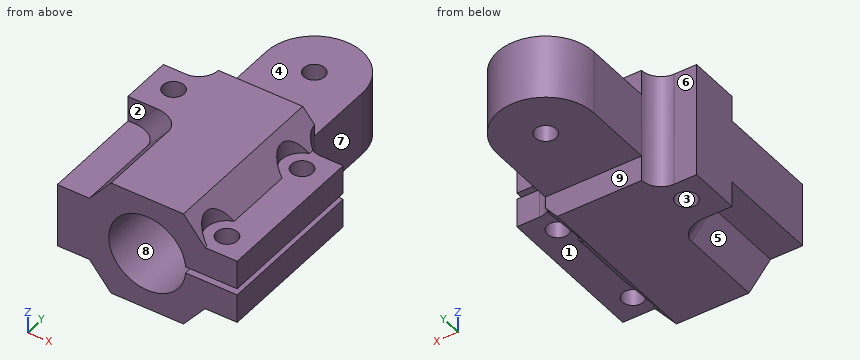
from build123d import *

# Parameters (mm, degrees)
F2_DEPTH        = 9
F3_R            = 6
F4_DEPTH        = 24
F6_DEPTH        = 45.3215080757
F7_DEPTH        = 16
F8_R            = 3
F10_DEPTH       = 21.501
F12_D           = 3.3
F12_START       = 4
F12_CBORE_D     = 6.5
F12_CBORE_DEPTH = 0
F14_D           = 3.3
F14_START       = 4
F14_CBORE_D     = 6.5
F14_CBORE_DEPTH = 0
F15_W           = 27
F15_H           = 1
F16_DEPTH       = 30


with BuildPart() as f2:
    # F1 (on Top) → F2 (new body, symmetric)
    with BuildSketch(Plane.XY):
        with BuildLine():
            ThreePointArc((-7.5, 0), (0, -7.5), (7.5, 0))
            ThreePointArc((7.5, 0), (0, 7.5), (-7.5, 0))
        make_face()
        with BuildLine():
            Line((7.5, -13.8205080757), (7.5, 0))
            ThreePointArc((7.5, 0), (0, -7.5), (-7.5, 0))
            Line((-7.5, 0), (-7.5, -13.8205080757))
            Line((-7.5, -13.8205080757), (-14, -13.8205080757))
            Line((-14, -13.8205080757), (-14, -37.8205080757))
            Line((-14, -37.8205080757), (14, -37.8205080757))
            Line((14, -37.8205080757), (14, -13.8205080757))
            Line((14, -13.8205080757), (7.5, -13.8205080757))
        make_face()
    extrude(amount=F2_DEPTH, both=True)

    # F3 (on face) → F4 (cut)
    with BuildSketch(Plane.XZ.offset(37.8205080757)):
        Circle(F3_R)
    extrude(amount=-F4_DEPTH, mode=Mode.SUBTRACT)

    # F5 (on face) → F6 (cut, through all)
    with BuildSketch(Plane.XZ.offset(37.8205080757)):
        Polygon((14, 9), (5.6436014753, 9), (9, 5), (14, 5), align=None)
        Polygon((14, -9), (14, -5), (9, -5), (5.6436014753, -9), align=None)
    extrude(amount=-F6_DEPTH, mode=Mode.SUBTRACT)

    # F5 (on face) → F7 (cut)
    with BuildSketch(Plane.XZ.offset(37.8205080757)):
        Polygon((-9, 5), (-5.6436014753, 9), (-14, 9), (-14, 5), align=None)
        Polygon((-9, -5), (-14, -5), (-14, -9), (-5.6436014753, -9), align=None)
    extrude(amount=-F7_DEPTH, mode=Mode.SUBTRACT)

    # F8
    f8_edges = [f2.edges().sort_by_distance(p)[0] for p in [
        (7.5, -13.820508, 0),
        (-7.5, -13.820508, 0),
        (-7.321801, -21.820508, 7),
        (-7.321801, -21.820508, -7),
    ]]
    fillet(f8_edges, radius=F8_R)

    # F9 (on face) → F10 (cut, through all)
    with BuildSketch(Plane.YZ.offset(7.5)):
        Polygon((9.9274870008, 9), (4.9396115625, 9), (-10.8205080757, 9), (-10.8205080757, 6.7876303889), (-10.8205080757, 5), (9.9274870008, 5), align=None)
        Polygon((9.9274870008, -5), (-10.8205080757, -5), (-10.8205080757, -6.7876303889), (-10.8205080757, -9), (9.9274870008, -9), align=None)
    extrude(amount=-F10_DEPTH, mode=Mode.SUBTRACT)

    # F12 (through all)
    # its depths count from where the whole tool has entered the part; down to there all is cleared
    with Locations(Plane.XY.offset(9)):
        with Locations((10, -34.3205080757, -F12_START), (10, -17.3205080757, -F12_START), (0, 0, -F12_START), (-10, -17.3205080757, 0)):
            CounterBoreHole(F12_D / 2, F12_CBORE_D / 2, F12_CBORE_DEPTH)

    # F14 (through all)
    # its depths count from where the whole tool has entered the part; down to there all is cleared
    with Locations(Plane(origin=(0, 0, -9), x_dir=(1, 0, 0), z_dir=(0, 0, -1)).offset(-F14_START)):
        with Locations((10, 34.3205080757), (10, 17.3205080757)):
            CounterBoreHole(F14_D / 2, F14_CBORE_D / 2, F14_CBORE_DEPTH)

    # F15 (on Right) → F16 (cut)
    with BuildSketch(Plane.YZ):
        with Locations((-24.3205080757, 0)):
            Rectangle(F15_W, F15_H)
    extrude(amount=F16_DEPTH, mode=Mode.SUBTRACT)


solid = f2.part
Model file for the job. Use its own axes, mm. Face numbers are marked on the shaded views. A direction names the side the tool comes from. Give positions to 0.01 mm unless a question says otherwise; leave off trailing zeros. Loops run counter-clockwise (first coordinate to the right, second up) from the corner with the lowest first, then second, coordinate; pieces in that order, holes last. Notation, with made-up numbers: (69, 73.25) - (91, 73.25) arc R17 cw to (91, 85.25) - close; hole circle Ø2 at (-10, 30.25). An arc over 180 degrees is marked (long way). Use one line per item in the form item = value.
(1) Cut at B-B (y = -18.5). Give the cut face in (x, z).
Determined:
outline = (-14, -9) - (-11.15, -9) - (-11.15, 9) - (-14, 9) - close; (-8.85, -9) - (5.64, -9) - (6.97, -7.42) - (6.97, -5) - (8.85, -5) - (8.85, -0.5) - (5.98, -0.5) arc R6 cw (long way) to (5.98, 0.5) - (8.85, 0.5) - (8.85, 5) - (6.97, 5) - (6.97, 7.42) - (5.64, 9) - (-8.85, 9) - close; (11.15, -5) - (14, -5) - (14, -0.5) - (11.15, -0.5) - close; (11.15, 0.5) - (14, 0.5) - (14, 5) - (11.15, 5) - close
(2) Pull direction Y, two halves, no side cores. Call the marked faces 1, 2, 3 and 4: pulls with the +Y half, pulls with the -Y half, needs draft (parallel to the pull), parting line crosses it, or undercut.
Determined:
face_1 = undercut
face_2 = pulls with the -Y half
face_3 = undercut
face_4 = needs draft
(3) Cut at D-D (z = -3). Give the cut face in (x, y).
Determined:
outline = (-14, -37.82) - (-5.2, -37.82) - (-5.2, -13.82) - (5.2, -13.82) - (5.2, -37.82) - (14, -37.82) - (14, -13.82) - (10.5, -13.82) arc R3 cw to (7.5, -10.82) - (7.5, 0) arc R7.5 ccw to (-7.5, 0) - (-7.5, -10.82) arc R3 cw to (-10.5, -13.82) - (-14, -13.82) - close; hole circle Ø3.3 at (-10, -17.32); hole circle Ø3.3 at (0, 0); hole circle Ø3.3 at (10, -34.32); hole circle Ø3.3 at (10, -17.32)
(4) Cut at C-C (x = 10). Give the cut face in (y, z), then the cut area to 3 significant figures.
Determined:
outline = (-37.82, -5) - (-35.97, -5) - (-35.97, -0.5) - (-37.82, -0.5) - close; (-37.82, 0.5) - (-35.97, 0.5) - (-35.97, 5) - (-37.82, 5) - close; (-32.67, -5) - (-18.97, -5) - (-18.97, -0.5) - (-32.67, -0.5) - close; (-32.67, 0.5) - (-18.97, 0.5) - (-18.97, 5) - (-32.67, 5) - close; (-15.67, -5) - (-13.78, -5) - (-13.78, -0.5) - (-15.67, -0.5) - close; (-15.67, 0.5) - (-13.78, 0.5) - (-13.78, 5) - (-15.67, 5) - close
area = 157 mm^2
(5) 3-axis set-ups, long thin cutter, end or side, ignore diameter. For the marked faces 5, 6, 7, 8 and 9: which of +Z, -Z, +X, -X, +Y, -Y reach the whole face in a straight line?
Determined:
face_5 = -Z, -X, -Y
face_6 = +Z, -Z, -X, +Y
face_7 = +Z, -Z, +X, +Y
face_8 = -Y
face_9 = -Z, +X, -X, +Y
(6) Drill centre lines: L1, parallel to Y at x = 10, z = -1.35; L2, parallel to Z at x = 0, y = -25.5; L3, parallel to Z at x = -9.5, y = -23.5. Where is each one in solid material? Low to high.
Determined:
L1 = -37.82 to -35.97, -32.67 to -18.97, -15.67 to -13.78
L2 = -9 to -6, 6 to 9
L3 = -5 to 5
(7) Cut at A-A (z = 0). Give the cut face in (x, y).
Determined:
outline = (-14, -37.82) - (-6, -37.82) - (-6, -13.82) - (0, -13.82) - (0, -10.82) - (7.5, -10.82) - (7.5, 0) arc R7.5 ccw to (-7.5, 0) - (-7.5, -10.82) arc R3 cw to (-10.5, -13.82) - (-14, -13.82) - close; hole circle Ø3.3 at (-10, -17.32); hole circle Ø3.3 at (0, 0)
(8) Drop flat-ended pins along their axis: P1, Ø2, axis at y = 0, z = 2.5, coming from the -X side; P2, Ø5, axis at x = 9, z = 1, coming from the +Y side; P3, Ø4, axis at x = 12, z = -3, coming from the +Y side. Give the stop position or say it passes through.
Determined:
P1 = -7.5
P2 = 3.74
P3 = -13.78
